CAD build for the part. Positions are in the model's coordinates, mm. Give positions to 0.01 mm unless a question says otherwise; leave off trailing zeros. Write each loop counter-clockwise with the first axis right and the second up, starting at its lowest first coordinate (ties: lowest second). Pieces come first, ordered by that corner, then holes. Notation, with made-up numbers: (77, -30.5) - (109, -30.5) arc R9 cw to (109, -14.5) - close; hole circle Ø5 at (85.5, 22.5). An arc over 180 degrees is marked (long way). Answer as a JSON object with one key per item and string values.
Autodesk Inventor part; units mm, degrees
ref_plane "YZ Plane" through (0, 0, 0) normal (1, 0, 0) x (0, 1, 0)
ref_plane "XZ Plane" through (0, 0, 0) normal (0, 1, 0) x (-1, 0, 0)
ref_plane "XY Plane" through (0, 0, 0) normal (0, 0, 1) x (1, 0, 0)
sketch "Boceto1" plane through (0, 0, 0) normal (0, 1, 0) x (-1, 0, 0)
  line L0 (0, 0) -> (1000, 0)
  line L1 (1000, 25) -> (1000, 1000)
  line L2 (975, 1000) -> (975, 25)
  line L3 (975, 25) -> (0, 25)
  line L4 (1025, 1000) -> (1025, 0)
  line L5 (1000, -25) -> (0, -25)
  line L6 (1025, 1000) -> (975, 1000)
  line L7 (0, -25) -> (0, 25)
  circle A0 centre (0, 0) radius 25
  circle A1 centre (1000, 1000) radius 25
  arc A2 (1000, -25) -> (1025, 0) centre (1000, 0) ccw
extrude "Extrusión1" add sketch "Boceto1" along normal blind 10
properties part number "suelo_pruebas"
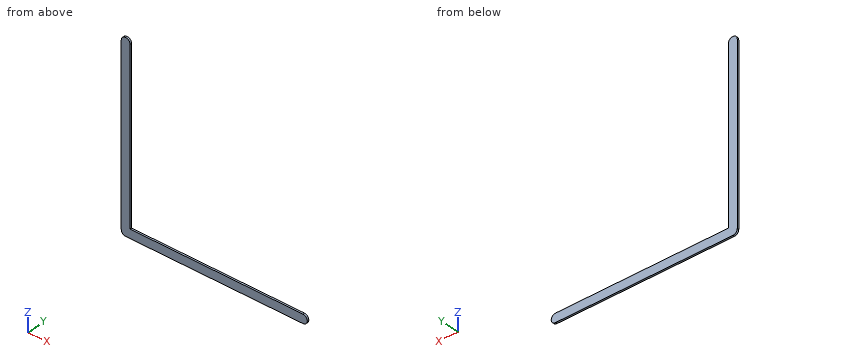
Item 1: Probe line 1 (X direction, y = 4.75, z = 665); line 2 (Z direction, x = -405.5, y = 1). List the from-to ranges inside material, lowest first. Write a range as from..to.
Entries:
{"line 1": "-1025..-975", "line 2": "-25..25"}
Item 2: Cut at C-C (z = 414.5). Give the cut face in (x, y), and give its area (3 significant figures).
Entries:
{"outline": "(-1025, 0) - (-975, 0) - (-975, 10) - (-1025, 10) - close", "area": "500 mm2"}
Item 3: Cut at A-A (y = 2.5). Give the cut face in (x, z), and give its area (3 significant figures).
Entries:
{"outline": "(-1025, 0) arc R25 ccw to (-1000, -25) - (0, -25) arc R25 ccw to (0, 25) - (-975, 25) - (-975, 1000) arc R25 ccw to (-1025, 1000) - close", "area": "102,000 mm2"}
Item 4: Flat gauge pins, fed straight in: P1, Ø4, axis at y = 7.5, z = 99, coming from the +X side; P2, Ø1.5, axis at x = -294, y = 6, coming from the +Z side. Where does each tip first touch, or does it go through?
Entries:
{"P1": "x = -975", "P2": "z = 25"}
Item 5: Cut at B-B (x = -748.5). Give the cut face in (y, z).
Entries:
{"outline": "(0, -25) - (10, -25) - (10, 25) - (0, 25) - close"}
